Build history of the part. All positions in model axes, mm. Give positions to 0.01 mm unless a question says otherwise; leave off trailing zeros. Order: outer loops, then holes, each group sorted by start corner. A loop starts at its lowest first (then second) coordinate and runs counter-clockwise, first axis right, second up. Notation, with made-up numbers: M 8,88.25 L 43,88.25 A27 cw 43,115.25 Z; hole C -17,69.25 d10. An arc over 180 degrees is marked long. One line per item, written item: value.
from build123d import *

# Parameters (mm, degrees)
ESQUISSE1_W             = 217.36
ESQUISSE1_H             = 12.11
BOSS_EXTRU_1_DEPTH      = 2
ESQUISSE2_W             = 8.5
ESQUISSE2_H             = 2.25
ESQUISSE2_W_2           = 10.5
ENL_V_MAT_EXTRU_1_DEPTH = 109.866916118
ESQUISSE4_W             = 2
ESQUISSE4_H             = 5.055
ENL_V_MAT_EXTRU_2_DEPTH = 109.866916118


with BuildPart() as part:
    # Esquisse1 → Boss.-Extru.1 (new body)
    with BuildSketch(Plane.XY):
        Rectangle(ESQUISSE1_W, ESQUISSE1_H)
    extrude(amount=BOSS_EXTRU_1_DEPTH)

    # Esquisse2 → Enlèv. mat.-Extru.1 (cut, through all)
    with BuildSketch(Plane(origin=(0, 0, 0), x_dir=(-1, 0, 0), z_dir=(0, 0, -1))):
        with Locations((-105.32, 5.18)):
            Rectangle(ESQUISSE2_W, ESQUISSE2_H)
        with Locations((-89.32, 5.18)):
            Rectangle(ESQUISSE2_W, ESQUISSE2_H)
        with Locations((-73.32, 5.18)):
            Rectangle(ESQUISSE2_W, ESQUISSE2_H)
        with Locations((-57.32, 5.18)):
            Rectangle(ESQUISSE2_W, ESQUISSE2_H)
        with Locations((-41.32, 5.18)):
            Rectangle(ESQUISSE2_W, ESQUISSE2_H)
        with Locations((-25.32, 5.18)):
            Rectangle(ESQUISSE2_W, ESQUISSE2_H)
        with Locations((-9.32, 5.18)):
            Rectangle(ESQUISSE2_W, ESQUISSE2_H)
        with Locations((6.68, 5.18)):
            Rectangle(ESQUISSE2_W, ESQUISSE2_H)
        with Locations((22.68, 5.18)):
            Rectangle(ESQUISSE2_W, ESQUISSE2_H)
        with Locations((38.68, 5.18)):
            Rectangle(ESQUISSE2_W, ESQUISSE2_H)
        with Locations((54.68, 5.18)):
            Rectangle(ESQUISSE2_W, ESQUISSE2_H)
        with Locations((70.68, 5.18)):
            Rectangle(ESQUISSE2_W, ESQUISSE2_H)
        with Locations((86.68, 5.18)):
            Rectangle(ESQUISSE2_W, ESQUISSE2_H)
        with Locations((103.68, 5.18)):
            Rectangle(ESQUISSE2_W_2, ESQUISSE2_H)
        with Locations((-86.68, -5.18)):
            Rectangle(ESQUISSE2_W, ESQUISSE2_H)
        with Locations((-70.68, -5.18)):
            Rectangle(ESQUISSE2_W, ESQUISSE2_H)
        with Locations((-54.68, -5.18)):
            Rectangle(ESQUISSE2_W, ESQUISSE2_H)
        with Locations((-38.68, -5.18)):
            Rectangle(ESQUISSE2_W, ESQUISSE2_H)
        with Locations((-22.68, -5.18)):
            Rectangle(ESQUISSE2_W, ESQUISSE2_H)
        with Locations((-6.68, -5.18)):
            Rectangle(ESQUISSE2_W, ESQUISSE2_H)
        with Locations((9.32, -5.18)):
            Rectangle(ESQUISSE2_W, ESQUISSE2_H)
        with Locations((25.32, -5.18)):
            Rectangle(ESQUISSE2_W, ESQUISSE2_H)
        with Locations((41.32, -5.18)):
            Rectangle(ESQUISSE2_W, ESQUISSE2_H)
        with Locations((57.32, -5.18)):
            Rectangle(ESQUISSE2_W, ESQUISSE2_H)
        with Locations((73.32, -5.18)):
            Rectangle(ESQUISSE2_W, ESQUISSE2_H)
        with Locations((89.32, -5.18)):
            Rectangle(ESQUISSE2_W, ESQUISSE2_H)
    extrude(amount=-ENL_V_MAT_EXTRU_1_DEPTH, mode=Mode.SUBTRACT)

    # Esquisse4 → Enlèv. mat.-Extru.2 (cut, through all)
    with BuildSketch(Plane(origin=(0, 0, 0), x_dir=(-1, 0, 0), z_dir=(0, 0, -1))):
        with Locations((107.68, 1.5275)):
            Rectangle(ESQUISSE4_W, ESQUISSE4_H)
    enl_v_mat_extru_2 = extrude(amount=-ENL_V_MAT_EXTRU_2_DEPTH, mode=Mode.SUBTRACT)

    # Symétrie1: Enlèv. mat.-Extru.2 across plane
    add(enl_v_mat_extru_2.mirror(Plane(origin=(0, 0, 0), x_dir=(0, 0, 1), z_dir=(1, 0, 0))), mode=Mode.SUBTRACT)


solid = part.part
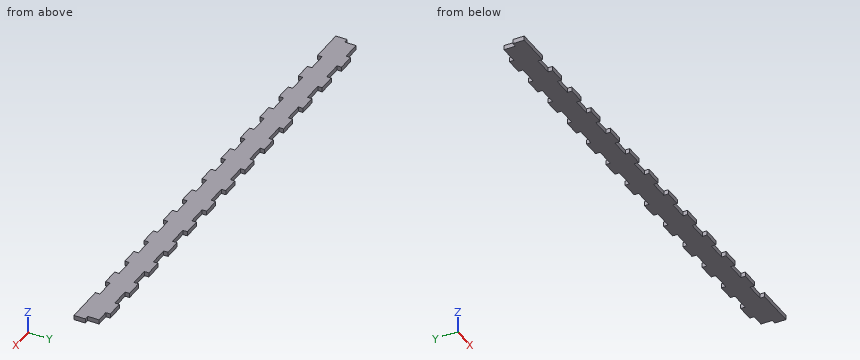
1) Pin check, flat tips, straight feed: pin 1 (1 mm diameter, centred on x = 57, z = 1, fed in from +Y) (3 decimals); pin 2 (0.6 mm diameter, centred on x = 25, z = 1, fed in from -Y) (3 decimals); pin 3 (0.6 mm diameter, centred on y = 5.5, z = 0.5, fed in from +X). Stop position of each tip, or through.
Check values:
pin 1: y = 4.055
pin 2: y = -4.055
pin 3: x = 101.07
2) Drill centre lines: probe 1 along Y at (x, z) = (-24, 0.75) (3 decimals); probe 2 along X at (y, z) = (0, 0.5); probe 3 along Y at (x, z) = (-84.5, 0.25) (3 decimals). Where is each one in solid material? Low to high. Write a range as from..to.
Check values:
probe 1: -4.055..4.055
probe 2: -106.68..106.68
probe 3: -6.055..4.055
3) Saw through at A-A, the plane x = -73. Write the cut outline in (y, z) (3 decimals).
Check values:
outline: M -4.055,0 L 4.055,0 L 4.055,2 L -4.055,2 Z
4) Saw through at B-B, the plane y = 2. Write the cut outline in (x, z).
Check values:
outline: M -106.68,0 L 106.68,0 L 106.68,2 L -106.68,2 Z
